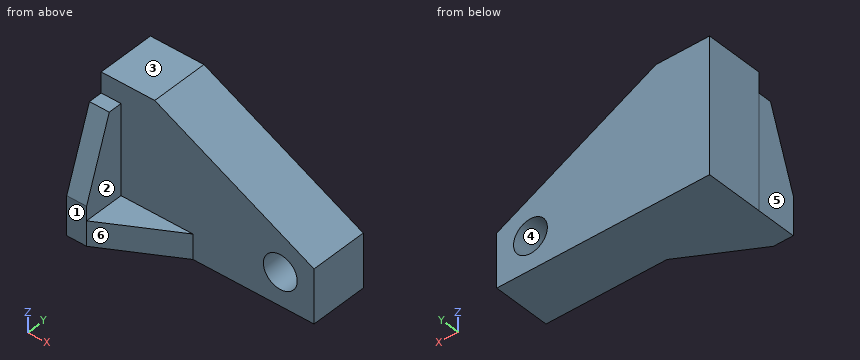
from build123d import *

# Parameters (mm, degrees)
F0_W      = 93.855083
F0_H      = 59.460982
F1_DEPTH  = 25.4
F3_DEPTH  = 25.4
F4_W      = 8.744262
F4_H      = 50.425246
F5_DEPTH  = 17.78
F7_DEPTH  = 25.4
F9_DEPTH  = 10.922
F10_R     = 7.465412
F11_DEPTH = 25.4


with BuildPart() as f1:
    # F0 (on Front) → F1 (new body)
    with BuildSketch(Plane.XZ):
        with Locations((6.412457, 0.437213)):
            Rectangle(F0_W, F0_H)
    extrude(amount=F1_DEPTH)

    # F2 (on face) → F3 (cut)
    with BuildSketch(Plane.XZ.offset(25.4)):
        Polygon((53.339999, 30.167704), (-16.905574, 30.167704), (53.339999, -5.683771), align=None)
    extrude(amount=-F3_DEPTH, mode=Mode.SUBTRACT)

    # F4 (on face) → F5 (join)
    with BuildSketch(Plane.XZ.offset(25.4)):
        with Locations((-36.142953, -4.080655)):
            Rectangle(F4_W, F4_H)
    extrude(amount=F5_DEPTH)

    # F6 (on face) → F7 (cut)
    with BuildSketch(Plane.YZ.offset(-31.770822)):
        Polygon((-43.18, -12.12093), (-31.462505, 21.131968), (-43.18, 21.131968), align=None)
    extrude(amount=-F7_DEPTH, mode=Mode.SUBTRACT)

    # F8 (on face) → F9 (join)
    with BuildSketch(Plane(origin=(0, 0, -29.293278), x_dir=(1, 0, 0), z_dir=(0, 0, -1))):
        Polygon((0, 25.4), (-31.770822, 43.18), (-31.770822, 25.4), align=None)
    extrude(amount=-F9_DEPTH)

    # F10 (on face) → F11 (cut)
    with BuildSketch(Plane.XZ.offset(25.4)):
        with Locations((38.474757, -14.719509)):
            Circle(F10_R)
    extrude(amount=-F11_DEPTH, mode=Mode.SUBTRACT)


solid = f1.part
Part model, mm, in its own coordinate system. Face numbers are marked on the shaded views. A direction names the side the tool comes from. Coordinates: 2 decimals unless noted, no trailing zeros. Loops run counter-clockwise (first coordinate to the right, second up) from the corner with the lowest first, then second, coordinate; pieces in that order, holes last. Notation, with made-up numbers: M 68.5,46 L 83.5,46 A23 ccw 83.5,77 Z; hole C 23.5,35.5 d3. An arc over 180 degrees is marked long. Use a Markdown table: item, result. Add a question column.
Q1. Cut at A-A (x = 40). Write the cut outline in (y, z), and give its area (3 significant figures).
Q2. Which spindle directions (+Z, -Z, +X, -X, +Y, -Y) get a long thin tool onto all of the face, cutting with end or side? Do the marked faces 1 and 2. Say none if no direction does.
Q3. Cut at D-D (x = -27). Write the cut outline in (y, z).
Q4. Probe L1, parallel to X at y = -39, z = -9.5; L2, parallel to Z at x = -19.5, y = -30.5; L3, parallel to Y at x = -29, z = 24. List the from-to ranges inside material, lowest first.
Q5. Mould opens along X. For the marked faces 3, 4, 5 and 6 say: +X half, -X half, draft (parallel to the pull), parting line (faces both ways), or undercut.
Q6. Cut at B-B (z = 15.5). Write the cut outline in (x, y).
Q7. Pin check, flat tips, straight feed: P1, Ø5, axis at y = -36, z = -14.5, coming from the +X side; P2, Ø9, axis at x = -18, y = -38.5, coming from the +Z side; P3, Ø5, axis at x = -38, y = -29.5, coming from the +Z side; P4, Ø13.5, axis at x = 38.47, z = -14.72, coming from the +Y side. Stop position of each tip, or through.
Q8. Cut at C-C (y = -11). Write the cut outline in (x, z).
Worked out:
| question | item | result |
|---|---|---|
| 1 | outline | M -25.4,-29.29 L 0,-29.29 L 0,-22.03 L -25.4,-22.03 Z; M -25.4,-7.41 L 0,-7.41 L 0,1.12 L -25.4,1.12 Z |
| 1 | area | 401 mm2 |
| 2 | face 1 | +Z, -Z, +X, -X, -Y |
| 2 | face 2 | +Z, +X, -Y |
| 3 | outline | M -40.51,-29.29 L 0,-29.29 L 0,30.17 L -25.4,30.17 L -25.4,-18.37 L -40.51,-18.37 Z |
| 4 | L1 | x = -40.52 to -31.77 |
| 4 | L2 | z = -29.29 to -18.37 |
| 4 | L3 | y = -25.4 to 0 |
| 5 | face 3 | draft |
| 5 | face 4 | undercut |
| 5 | face 5 | -X half |
| 5 | face 6 | +X half |
| 6 | outline | M -40.52,-33.45 L -31.77,-33.45 L -31.77,-25.4 L 11.83,-25.4 L 11.83,0 L -40.52,0 Z |
| 7 | P1 | stops at x = -31.77 |
| 7 | P2 | stops at z = -18.37 |
| 7 | P3 | stops at z = 21.13 |
| 7 | P4 | passes through |
| 8 | outline | M -40.52,-29.29 L 53.34,-29.29 L 53.34,-5.68 L -16.91,30.17 L -40.52,30.17 Z; hole C 38.47,-14.72 d14.93 |
